from build123d import *

# Parameters (mm, degrees)
CROQUIS1_R              = 12
SALIENTE_EXTRUIR1_DEPTH = 2.5
CROQUIS2_R              = 5
SALIENTE_EXTRUIR2_DEPTH = 5
CROQUIS3_R              = 3.1
CORTAR_EXTRUIR1_DEPTH   = 4.2
CROQUIS4_R              = 1.5
CORTAR_EXTRUIR2_DEPTH   = 4
CROQUIS5_R              = 1.5
SALIENTE_EXTRUIR3_DEPTH = 2.5
CROQUIS6_R              = 0.75
CORTAR_EXTRUIR3_DEPTH   = 2


with BuildPart() as part:
    # Croquis1 → Saliente-Extruir1 (new body)
    with BuildSketch(Plane.XY):
        Circle(CROQUIS1_R)
    extrude(amount=SALIENTE_EXTRUIR1_DEPTH)

    # Croquis2 → Saliente-Extruir2 (add)
    with BuildSketch(Plane(origin=(0, 0, 0), x_dir=(-1, 0, 0), z_dir=(0, 0, -1))):
        Circle(CROQUIS2_R)
    extrude(amount=SALIENTE_EXTRUIR2_DEPTH)

    # Croquis3 → Cortar-Extruir1 (cut)
    with BuildSketch(Plane(origin=(0, 0, -5), x_dir=(-1, 0, 0), z_dir=(0, 0, -1))):
        Circle(CROQUIS3_R)
    extrude(amount=-CORTAR_EXTRUIR1_DEPTH, mode=Mode.SUBTRACT)

    # Croquis4 → Cortar-Extruir2 (cut)
    with BuildSketch(Plane.XY.offset(2.5)):
        Circle(CROQUIS4_R)
    extrude(amount=-CORTAR_EXTRUIR2_DEPTH, mode=Mode.SUBTRACT)

    # Croquis5 → Saliente-Extruir3 (add)
    with BuildSketch(Plane.XY.offset(2.5)):
        with Locations((9.5, 0)):
            Circle(CROQUIS5_R)
        with Locations((-9.5, 0)):
            Circle(CROQUIS5_R)
    extrude(amount=SALIENTE_EXTRUIR3_DEPTH)

    # Croquis6 → Cortar-Extruir3 (cut)
    with BuildSketch(Plane(origin=(0, 0, 0), x_dir=(-1, 0, 0), z_dir=(0, 0, -1))):
        with Locations((-9.5, 0)):
            Circle(CROQUIS6_R)
        with Locations((9.5, 0)):
            Circle(CROQUIS6_R)
    extrude(amount=-CORTAR_EXTRUIR3_DEPTH, mode=Mode.SUBTRACT)


solid = part.part
Model file for the job. Use its own axes, mm. A direction names the side the tool comes from. Coordinates: 2 decimals unless noted, no trailing zeros. Order: outer loops, then holes, each group sorted by start corner. A loop starts at its lowest first (then second) coordinate and runs counter-clockwise, first axis right, second up. Notation, with made-up numbers: M -17.75,0 L -12.75,0 A28 cw -12.75,30 Z; hole C 17.5,68.25 d11. An arc over 180 degrees is marked long. Return JSON: item names as keys, results as strings.
1. Tool access for faces 1 (the face through (8, 0, 4)), 2 (the face through (-1.43, -2.75, -2.93)), 3 (the face through (-1.5, 0.07, 0.87)): list every direction of +Z, -Z, +X, -X, +Y, -Y with a clear straight run to the whole face (end or side of a thin tool).
Ans:
{"face 1": "+Z", "face 2": "-Z", "face 3": "+Z, -Z"}
2. Pull direction Y, two halves, no side cores. Call faces 4 (the face through (0.1, -3.3, -5)), 5 (the face through (10, 0, 2)), 6 (the face through (-11.99, 0.53, 1.23)), 7 (the face through (-8.75, 0.03, 0.99)): +Y half, -Y half, draft (parallel to the pull), parting line (faces both ways), or undercut.
Ans:
{"face 4": "draft", "face 5": "undercut", "face 6": "parting line", "face 7": "undercut"}
3. Drill centre lines: probe 1 along Y at (x, z) = (0, 0.1); probe 2 along Z at (x, y) = (-3.5, 10.5); probe 3 along Y at (x, z) = (-2.25, -2). Where is each one in solid material? Low to high.
Ans:
{"probe 1": "-12 to -1.5, 1.5 to 12", "probe 2": "0 to 2.5", "probe 3": "-4.47 to -2.13, 2.13 to 4.47"}
4. Saw through at D-D (z = 1). Give the cut face in (x, y), and give its area (3 significant figures).
Ans:
{"outline": "C 0,0 d24; hole C -9.5,0 d1.5; hole C 0,0 d3; hole C 9.5,0 d1.5", "area": "442 mm^2"}
5. Saw through at A-A (x = 0). Give the cut face in (y, z).
Ans:
{"outline": "M -12,0 L -5,0 L -5,-5 L -3.1,-5 L -3.1,-0.8 L -1.5,-0.8 L -1.5,2.5 L -12,2.5 Z; M 1.5,-0.8 L 3.1,-0.8 L 3.1,-5 L 5,-5 L 5,0 L 12,0 L 12,2.5 L 1.5,2.5 Z"}
6. Saw through at C-C (z = -0.5). Give the cut face in (x, y).
Ans:
{"outline": "C 0,0 d10; hole C 0,0 d3"}
7. Flat gauge pins, fed straight in: pin 1 (1.9 mm diameter, centred on x = -1, y = -0.5, fed in from -Z); pin 2 (1.2 mm diameter, centred on x = 10, y = 0, fed in from -Z); pin 3 (5 mm diameter, centred on x = -3.5, z = -2, fed in from +Y). Where does each tip first touch, or does it go through?
Ans:
{"pin 1": "z = -0.8", "pin 2": "z = 0", "pin 3": "y = 11.83"}
